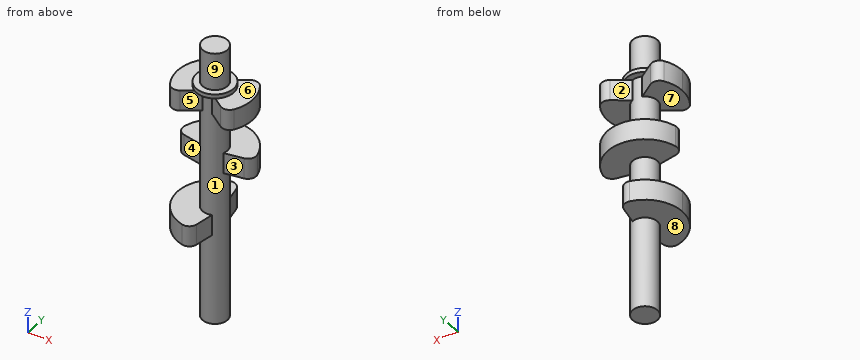
from build123d import *

# Parameters (mm, degrees)
SKETCH_2_R       = 1.5
SHAFT_DEPTH      = 33.5
EXCENTRIC1_DEPTH = 2.5
EXTRUDE_3_DEPTH  = 2.5
EXTRUDE_4_DEPTH  = 2.5
FILLET_1_R       = 1
SKETCH_7_R       = 2.25
EXTRUDE_5_DEPTH  = 0.5


with BuildPart() as part:
    # Эскиз2 → shaft (new body)
    with BuildSketch(Plane.XY):
        Circle(SKETCH_2_R)
    extrude(amount=SHAFT_DEPTH)

    # Эскиз3 → excentric1 (add)
    with BuildSketch(Plane(origin=(0, 0, 11), x_dir=(-1, 0, 0), z_dir=(0, 0, -1))):
        with BuildLine():
            ThreePointArc((4.5, 0), (3.181980515, 3.181980515), (0, 4.5))
            Line((0, 4.5), (-0.574025149, 1.385819299))
            ThreePointArc((-0.574025149, 1.385819299), (0.83335535, 1.247204418), (1.5, 0))
            ThreePointArc((1.5, 0), (0.83335535, -1.247204418), (-0.574025149, -1.385819299))
            Line((-0.574025149, -1.385819299), (0, -4.5))
            ThreePointArc((0, -4.5), (3.181980515, -3.181980515), (4.5, 0))
        make_face()
    extrude(amount=-EXCENTRIC1_DEPTH)

    # excentric2sketch → Бобышка-Вытянуть3 (add)
    with BuildSketch(Plane(origin=(0, 0, 18.5), x_dir=(-1, 0, 0), z_dir=(0, 0, -1))):
        with BuildLine():
            ThreePointArc((4.5, 0), (0, 4.5), (-4.5, 0))
            Line((-4.5, 0), (-1.385819299, -0.574025149))
            ThreePointArc((-1.385819299, -0.574025149), (-0.292635483, 1.471177921), (1.5, 0))
            ThreePointArc((1.5, 0), (1.471177921, -0.292635483), (1.385819299, -0.574025149))
            Line((1.385819299, -0.574025149), (4.5, 0))
        make_face()
    extrude(amount=-EXTRUDE_3_DEPTH)

    # excentric3sketch → Бобышка-Вытянуть4 (add)
    with BuildSketch(Plane(origin=(0, 0, 26), x_dir=(-1, 0, 0), z_dir=(0, 0, -1))):
        with BuildLine():
            Line((-0.574025149, 1.385819299), (-3.181980515, 3.181980515))
            ThreePointArc((-3.181980515, 3.181980515), (-4.5, 0), (-3.181980515, -3.181980515))
            Line((-3.181980515, -3.181980515), (-0.574025149, -1.385819299))
            ThreePointArc((-0.574025149, -1.385819299), (-1.5, 0), (-0.574025149, 1.385819299))
        make_face()
        with BuildLine():
            ThreePointArc((4.5, 0), (4.157457896, 1.722075446), (3.181980515, 3.181980515))
            Line((3.181980515, 3.181980515), (0.574025149, 1.385819299))
            ThreePointArc((0.574025149, 1.385819299), (1.247204418, 0.83335535), (1.5, 0))
            ThreePointArc((1.5, 0), (1.247204418, -0.83335535), (0.574025149, -1.385819299))
            Line((0.574025149, -1.385819299), (3.181980515, -3.181980515))
            ThreePointArc((3.181980515, -3.181980515), (4.157457896, -1.722075446), (4.5, 0))
        make_face()
    extrude(amount=-EXTRUDE_4_DEPTH)

    # Скругление1
    fillet_1_edges = [part.edges().sort_by_distance(p)[0] for p in [
        (4.5, 0, 19.75),
        (-4.5, 0, 19.75),
        (3.181980515, -3.181980515, 27.25),
        (3.181980515, 3.181980515, 27.25),
        (-3.181980515, 3.181980515, 27.25),
        (-3.181980515, -3.181980515, 27.25),
        (0, 4.5, 12.25),
        (0, -4.5, 12.25),
    ]]
    fillet(fillet_1_edges, radius=FILLET_1_R)

    # Эскиз7 → Бобышка-Вытянуть5 (add)
    with BuildSketch(Plane.XY.offset(28.5)):
        Circle(SKETCH_7_R)
    extrude(amount=EXTRUDE_5_DEPTH)


solid = part.part
Here's how the part is built. I have some questions about the finished solid (model axes, mm). Face numbers are marked on the shaded views. A direction names the side the tool comes from. Round coordinates to 2 decimals unless told otherwise and drop trailing zeros. Write each loop counter-clockwise with the first axis right and the second up, starting at its lowest first coordinate (ties: lowest second). Pieces come first, ordered by that corner, then holes.
1. Suppose I cut it at B-B (z = 27). List the corners of the cut face in (x, y) for me.
2. If we mould it in two halves opening along Z, with no side actions, what happens to the marked faces 6, 7, 8 and 9? For each: released by +Z, released by -Z, zero draft, split by the parting line, or undercut.
3. Suppose I cut it at A-A (x = 3.25). List the corners of the cut face in (y, z) for me, and give its area (3 significant figures).
4. Suppose I cut it at C-C (x = -3.25). List the corners of the cut face in (y, z) for me, and give its area (3 significant figures).
5. I need wall thicknesses on L1, parallel to Z at x = -3.5, y = 2.5; L2, parallel to Z at x = 2.75, y = 0.75; L3, parallel to Z at x = 1, y = 1.75. Which ranges of each line are inside material? Lowest first, please.
6. Will these pins go through, and if not, where does the flat tip stop? pin 1 Ø4 at (y, z) = (-3, 17.5) entering from +X; pin 2 Ø3 at (y, z) = (-3.5, 24.5) entering from +X; pin 3 Ø1 at (x, z) = (0.5, 26.5) entering from +Y; pin 4 Ø1.5 at (x, y) = (-3.5, 3) entering from -Z.
7. Suppose I cut it at D-D (z = 3). List the corners of the cut face in (x, y) for me, and give its area (3 significant figures).
8. For the marked faces 1, 2, 3, 4 and 5, which set-ups out of +Z, -Z, +X, -X, +Y, -Y let a thin tool reach every point of the face, with its end or its side?
Answer sheet:
1. outline: (-3.84, -2.35) arc R1 ccw to (-2.42, -2.65) - (-0.57, -1.39) arc R1.5 ccw to (0.57, -1.39) - (2.42, -2.65) arc R1 ccw to (3.84, -2.35) arc R4.5 ccw to (3.84, 2.35) arc R1 ccw to (2.42, 2.65) - (0.57, 1.39) arc R1.5 ccw to (-0.57, 1.39) - (-2.42, 2.65) arc R1 ccw to (-3.84, 2.35) arc R4.5 ccw to start
2. face 6: released by +Z
2. face 7: undercut
2. face 8: released by -Z
2. face 9: zero draft
3. outline: (-2.79, 26) - (2.79, 26) - (2.79, 28.5) - (-2.79, 28.5) - close; (-0.23, 18.5) - (3.11, 18.5) - (3.11, 21) - (-0.23, 21) - close
3. area: 22.3 mm2
4. outline: (-3.11, 11) - (3.11, 11) - (3.11, 13.5) - (-3.11, 13.5) - close; (-2.79, 26) - (2.79, 26) - (2.79, 28.5) - (-2.79, 28.5) - close; (-0.23, 18.5) - (3.11, 18.5) - (3.11, 21) - (-0.23, 21) - close
4. area: 37.9 mm2
5. L1: z = 11 to 13.5, 18.5 to 21, 26 to 28.5
5. L2: z = 18.5 to 21, 26 to 28.5
5. L3: z = 18.5 to 21, 28.5 to 29
6. pin 1: stops at x = 1.12
6. pin 2: passes through
6. pin 3: stops at y = 1.68
6. pin 4: stops at z = 11
7. outline: circle Ø3 at (0, 0)
7. area: 7.07 mm2
8. face 1: none
8. face 2: +Y
8. face 3: -Z, +X, -Y
8. face 4: -X, -Y
8. face 5: -Y
